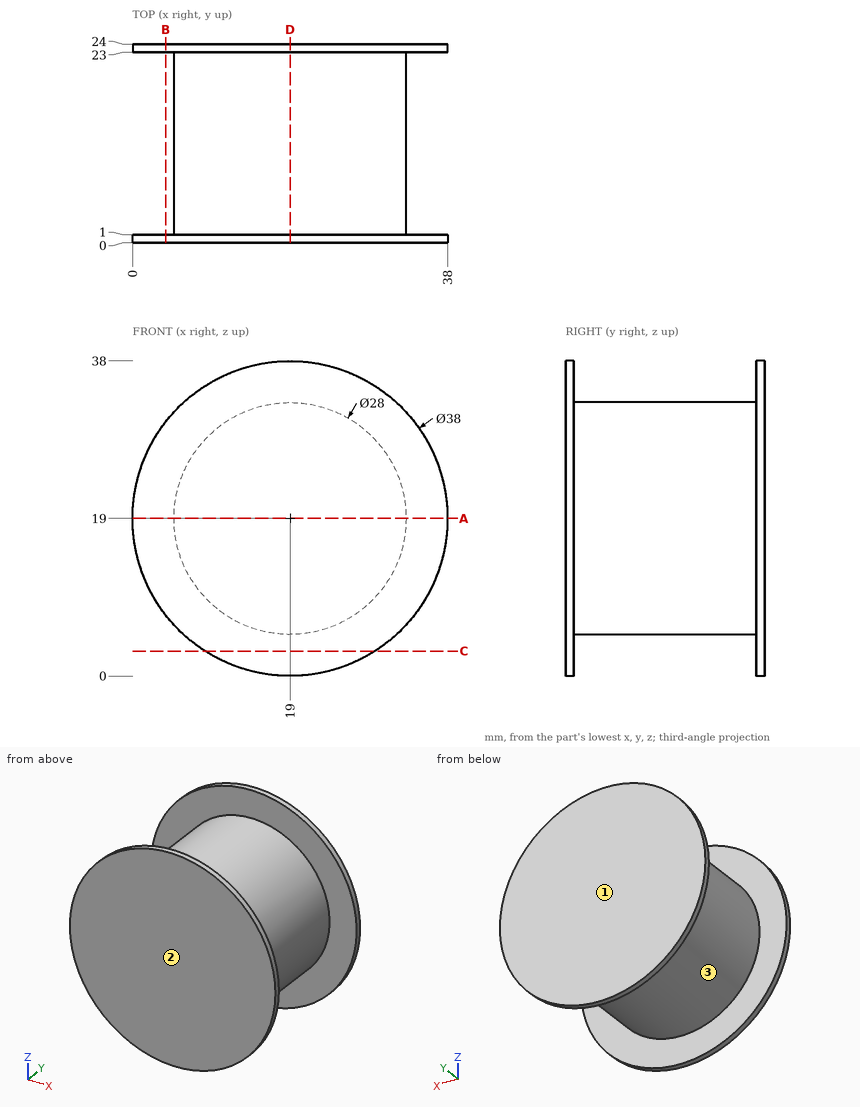
Geometry: see drawing. Coordinates: mm, zero at the bounding-box minimum. Give positions to 0.01 mm unless a question says otherwise; leave off trailing zeros. Loops run counter-clockwise (first coordinate to the right, second up) from the corner with the lowest first, then second, coordinate; pieces in that order, holes last. Notation, with made-up numbers: M -34,18.25 L -11,18.25 A8 cw -11,33.25 Z; hole C 21,12 d1. An arc over 180 degrees is marked long. Answer as CSV lines item,"result". Start each with the question number.
1. Section A-A on z = 19. Return loops of the section in (x, y).
2. Section C-C on z = 3. Return loops of the section in (x, y), plus the area to 3 significant figures.
3. Line query: L1, parallel to Y at x = 4, z = 29; L2, parallel to X at y = 18, z = 18.5; L3, parallel to Z at x = 19, y = 18.5. Output: solid intervals per line, ascending.
4. Section B-B on x = 4. Return loops of the section in (y, z).
5. Section D-D on x = 19. Return loops of the section in (y, z), plus the area to 3 significant figures.
6. Pin query (flat end, axial travel): P1, Ø12, axis at y = 10, z = 5.5, coming from the -X side; P2, Ø8, axis at y = 18, z = 8.5, coming from the +X side; P3, Ø8, axis at x = 4.5, y = 8.5, coming from the -Z side. Return the tip coordinate at first contact, or that it passes through.
7. Pull-direction query (Y, two-part tool) for the marked faces 1, 2 and 3; classes: released by +Y, released by -Y, zero draft, split by the parting line, or undercut.
Computed values:
1,outline,"M 0,0 L 38,0 L 38,1 L 33,1 L 33,23 L 38,23 L 38,24 L 0,24 L 0,23 L 5,23 L 5,1 L 0,1 Z"
2,outline,"M 8.75,0 L 29.25,0 L 29.25,1 L 8.75,1 Z; M 8.75,23 L 29.25,23 L 29.25,24 L 8.75,24 Z"
2,area,"41.0 mm²"
3,L1,"y = 0 to 1, 23 to 24"
3,L2,"x = 5.01 to 32.99"
3,L3,"z = 5 to 33"
4,outline,"M 0,7.34 L 1,7.34 L 1,30.66 L 0,30.66 Z; M 23,7.34 L 24,7.34 L 24,30.66 L 23,30.66 Z"
5,outline,"M 0,0 L 1,0 L 1,5 L 23,5 L 23,0 L 24,0 L 24,38 L 23,38 L 23,33 L 1,33 L 1,38 L 0,38 Z"
5,area,"692 mm²"
6,P1,"stops at x = 7.18"
6,P2,"stops at x = 31.4"
6,P3,"stops at z = 9.74"
7,face 1,"released by +Y"
7,face 2,"released by -Y"
7,face 3,"undercut"
